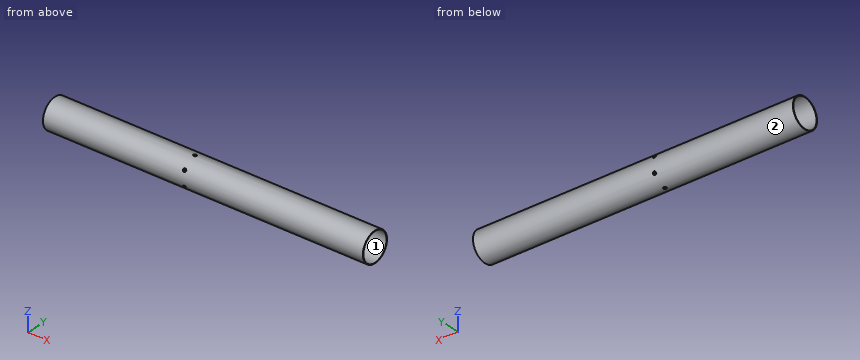
```python
from build123d import *

# Parameters (mm, degrees)
SKETCH1_R           = 28.4734
SKETCH1_R_2         = 27.3304
BOSS_EXTRUDE1_DEPTH = 609.6
CIRPATTERN1_COUNT   = 6


# Read off the part's stored shape, not the designer's step: CSK for #5 Flat Head Machine Screw1
with BuildPart() as part:
    # Sketch1 → Boss-Extrude1 (new body)
    with BuildSketch(Plane(origin=(0, 0, 0), x_dir=(0, 0, -1), z_dir=(1, 0, 0))):
        with Locations(Location((0, 0, 0), (0, 0, 180))):
            Circle(SKETCH1_R)
        with Locations(Location((0, 0, 0), (0, 0, 180))):
            Circle(SKETCH1_R_2, mode=Mode.SUBTRACT)
    extrude(amount=BOSS_EXTRUDE1_DEPTH)

    # CSK for #5 Flat Head Machine Screw1 outl → CSK for #5 Flat Head Machine Screw1 (revolve, cut)
    with BuildSketch(Plane(origin=(266.7, 0, 0), x_dir=(1, 0, 0), z_dir=(0, -1, 0))):
        Polygon((3.001715891, 28.473440077), (0, 28.473440077), (0, 27.260877218), (1.947651078, 27.260877218), align=None)
    csk_for_5_flat_head_machine_screw1 = revolve(axis=Axis((266.7, 0, 0), (0, 0, 1)), mode=Mode.SUBTRACT)

    # CirPattern1: CSK for #5 Flat Head Machine Screw1 ×6 about axis
    cirpattern1_axis = Axis((609.6, 0, 0), (-1, 0, 0))
    for i in range(1, CIRPATTERN1_COUNT):
        add(csk_for_5_flat_head_machine_screw1.rotate(cirpattern1_axis, i * 360 / CIRPATTERN1_COUNT), mode=Mode.SUBTRACT)


solid = part.part
```
Read the model definition and answer for the solid it produces. Units are mm, in the model's axes. Face numbers are marked on the shaded views. Coordinates: 2 decimals unless noted, no trailing zeros. Write each loop counter-clockwise with the first axis right and the second up, starting at its lowest first coordinate (ties: lowest second). Pieces come first, ordered by that corner, then holes. Notation, with made-up numbers: (-34, 8) -> (-25, 8) arc R13 ccw to (-25, 31) -> close; hole circle Ø3 at (-6.75, -3.75). An arc over 180 degrees is marked (long way). Write item = value, one per line.
(1) For a pull along Y with two mould halves and no side action, classify the marked faces 1 and 2 as +Y half, -Y half, draft (parallel to the pull), parting line (faces both ways), or undercut.
From the geometry:
face_1 = undercut
face_2 = parting line
(2) Section B-B on y = 15.5 is taken. Write down the section's boundary in (x, z).
From the geometry:
outline = (0, -23.88) -> (609.6, -23.88) -> (609.6, -22.51) -> (0, -22.51) -> close; (0, 22.51) -> (609.6, 22.51) -> (609.6, 23.88) -> (0, 23.88) -> close
(3) Section A-A on z = 0 is taken. Write down the section's boundary in (x, y).
From the geometry:
outline = (0, -28.47) -> (609.6, -28.47) -> (609.6, -27.33) -> (0, -27.33) -> close; (0, 27.33) -> (609.6, 27.33) -> (609.6, 28.47) -> (0, 28.47) -> close
(4) Straight lines are drawn through the part: L1, parallel to Y at x = 299, z = 0; L2, parallel to Y at x = 196, z = -2; L3, parallel to Z at x = 34.5, y = -4. For each, find the intervals that lie inside material, in ascending order. Write a range as from..to.
From the geometry:
L1 = -28.47..-27.33, 27.33..28.47
L2 = -28.4..-27.26, 27.26..28.4
L3 = -28.19..-27.04, 27.04..28.19
(5) Given pin 1 Ø10 at (x, y) = (140.5, 11.5) entering from +Z; pin 2 Ø5 at (x, y) = (145, 10) entering from -Z; pin 3 Ø12 at (x, z) = (179, 4.5) entering from +Y; pin 4 Ø10 at (x, y) = (331, 5) entering from +Z, each flat-ended and moving along its own axis, determine where each tip first touches the part or whether it passes through.
From the geometry:
pin_1 = 27.72
pin_2 = -27.47
pin_3 = 28.47
pin_4 = 28.47
(6) Section C-C on x = 501 is taken. Write down the section's boundary in (y, z).
From the geometry:
outline = circle Ø56.95 at (0, 0); hole circle Ø54.66 at (0, 0)
